```python
from build123d import *

# Parameters (mm, degrees)
CROQUIS1_R              = 5.9
SALIENTE_EXTRUIR1_DEPTH = 4.8
CROQUIS2_R              = 3.9
SALIENTE_EXTRUIR2_DEPTH = 13.4
CROQUIS3_R              = 2.5
CORTAR_EXTRUIR1_DEPTH   = 14.4
CHAFL_N1_SIZE           = 0.1
CROQUIS4_R              = 2.5
CROQUIS5_R              = 1.5
CORTAR_EXTRUIR2_DEPTH   = 6.9


with BuildPart() as part:
    # Croquis1 → Saliente-Extruir1 (new body)
    with BuildSketch(Plane(origin=(0, 0, 0), x_dir=(1, 0, 0), z_dir=(0, 1, 0))):
        Circle(CROQUIS1_R)
    extrude(amount=SALIENTE_EXTRUIR1_DEPTH)

    # Croquis2 → Saliente-Extruir2 (add)
    with BuildSketch(Plane(origin=(0, 0, 0), x_dir=(1, 0, 0), z_dir=(0, 1, 0))):
        Circle(CROQUIS2_R)
    extrude(amount=SALIENTE_EXTRUIR2_DEPTH)

    # Croquis3 → Cortar-Extruir1 (cut, through all)
    with BuildSketch(Plane(origin=(0, 13.4, 0), x_dir=(1, 0, 0), z_dir=(0, 1, 0))):
        Circle(CROQUIS3_R)
    extrude(amount=-CORTAR_EXTRUIR1_DEPTH, mode=Mode.SUBTRACT)

    # Chaflán1
    chafl_n1_edges = [part.edges().sort_by_distance(p)[0] for p in [
        (-2.5, 0, 0),
        (-2.5, 13.4, 0),
        (-5.9, 0, 0),
        (-5.9, 4.8, 0),
        (-3.9, 13.4, 0),
    ]]
    chamfer(chafl_n1_edges, length=CHAFL_N1_SIZE)

    # Croquis4 → Cortar-Revolución2 (revolve, cut)
    with BuildSketch(Plane(origin=(0, 0, 0), x_dir=(0, 0, -1), z_dir=(1, 0, 0))):
        with Locations((-5.6, 10.1)):
            Circle(CROQUIS4_R)
    revolve(axis=Axis((0, 13.979474026, 0), (0, -1, 0)), mode=Mode.SUBTRACT)

    # Croquis5 → Cortar-Extruir2 (cut, through all)
    with BuildSketch(Plane.XY):
        with Locations((0, 2.4)):
            Circle(CROQUIS5_R)
    extrude(amount=-CORTAR_EXTRUIR2_DEPTH, mode=Mode.SUBTRACT)


solid = part.part
```
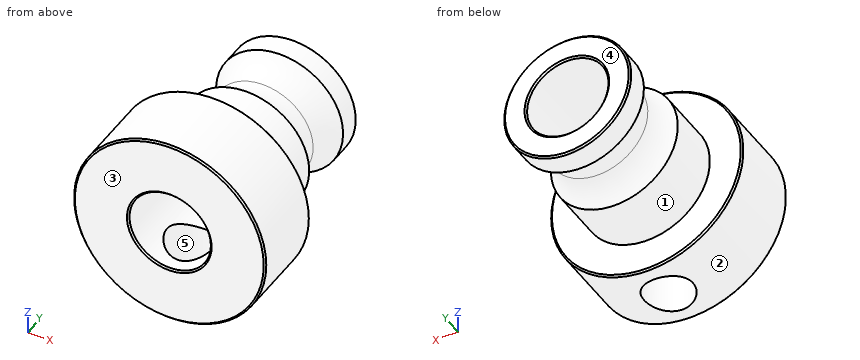
Input: part model. Units: mm. Frame: model coordinates. Face numbers are marked on the shaded views. A direction names the side the tool comes from. Coordinates: 2 decimals unless noted, no trailing zeros. Write each loop counter-clockwise with the first axis right and the second up, starting at its lowest first coordinate (ties: lowest second). Pieces come first, ordered by that corner, then holes. Notation, with made-up numbers: (6.25, 64.5) -> (63.25, 64.5) arc R17 cw to (63.25, 97.5) -> close; hole circle Ø9 at (-14, 55). An arc over 180 degrees is marked (long way). Answer as a JSON object with one key per item and string values.
1. Section A-A on x = 0. Count the separate pieces of the cut face and the enclosed holes in it, then the cut area to 3 significant figures.
Result set:
{"separate pieces": "3", "enclosed holes": "0", "area": "42.4 mm2"}
2. Section C-C on y = 6. Return the cut outline in (x, z), then the cut area to 3 significant figures.
Result set:
{"outline": "circle Ø7.8 at (0, 0); hole circle Ø5 at (0, 0)", "area": "28.1 mm2"}
3. Access query for the marked faces 1 and 2. Directions: +Z, -Z, +X, -X, +Y, -Y. A direction counts if a zero-diameter tool reaches every point of the face in a straight line with its end or side. Return the directions, or none.
Result set:
{"face 1": "+Y", "face 2": "+Y, -Y"}
4. First-contact query: P1, Ø1, axis at y = 2.5, z = 1, coming from the +X side; P2, Ø6.5, axis at x = 0, z = 0, coming from the +Y side; P3, Ø6, axis at x = 0.5, y = 8, coming from the +Z side. Flat tips, straight axial feed; report the tip coordinate or a pass-through.
Result set:
{"P1": "stops at x = 5.88", "P2": "stops at y = 13.4", "P3": "stops at z = 3.9"}
5. Section D-D on y = 2.4. Return the cut outline in (x, z).
Result set:
{"outline": "(-1.5, -5.71) -> (-1.5, -2) arc R2.5 cw (long way) to (1.5, -2) -> (1.5, -5.71) arc R5.9 ccw (long way) to start"}
6. Material intervals for line 1 (Z direction, x = 0, y = 5.75); line 2 (Y direction, x = 0, z = -4.2), sorted ascending. Write a range as from..to.
Result set:
{"line 1": "z = -3.9..-2.5, 2.5..3.9", "line 2": "y = 0..0.9, 3.9..4.8"}
7. Section B-B on z = 0. Return the cut outline in (x, y).
Result set:
{"outline": "(-5.9, 0.1) -> (-5.8, 0) -> (-2.6, 0) -> (-2.5, 0.1) -> (-2.5, 13.3) -> (-2.6, 13.4) -> (-3.8, 13.4) -> (-3.9, 13.3) -> (-3.9, 11.93) arc R2.5 cw to (-3.9, 8.27) -> (-3.9, 4.8) -> (-5.8, 4.8) -> (-5.9, 4.7) -> close; (2.5, 0.1) -> (2.6, 0) -> (5.8, 0) -> (5.9, 0.1) -> (5.9, 4.7) -> (5.8, 4.8) -> (3.9, 4.8) -> (3.9, 8.27) arc R2.5 cw to (3.9, 11.93) -> (3.9, 13.3) -> (3.8, 13.4) -> (2.6, 13.4) -> (2.5, 13.3) -> close"}
8. Mould query, pull axis Y, two halves, no side actions, for the marked faces 3, 4 and 5. Classes: released by +Y, released by -Y, zero draft, split by the parting line, or undercut.
Result set:
{"face 3": "released by -Y", "face 4": "released by +Y", "face 5": "undercut"}
